```python
from build123d import *

# Parameters (mm, degrees)
SKETCH1_W                    = 50.8
SKETCH1_H                    = 40
BASE_FLANGE1_DEPTH           = 0.635
EDGE_FLANGE1_STRIP_W         = 4.54
EDGE_FLANGE1_STRIP_H         = 0.635
EDGE_FLANGE1_STRIP_CUT_DEPTH = 50.8
EDGE_FLANGE1_DEPTH           = 50.8
SKETCH9_R                    = 8.75
CUT_EXTRUDE1_DEPTH           = 35.48419928
SKETCH10_R                   = 2.65
CUT_EXTRUDE2_DEPTH           = 49.360761212


# Sheet-metal steps are written as plain solids
with BuildPart() as part:
    # Sketch1 → Base-Flange1 (new body)
    with BuildSketch(Plane(origin=(0, 0, 0), x_dir=(0, 0, -1), z_dir=(1, 0, 0))):
        Rectangle(SKETCH1_W, SKETCH1_H)
    extrude(amount=-BASE_FLANGE1_DEPTH)

    # Edge-Flange1 strip (across the edge) → Edge-Flange1 strip cut (cut)
    with BuildSketch(Plane(origin=(-0.635, -20, -25.4), x_dir=(0, 1, 0), z_dir=(0, 0, 1))):
        with Locations((-0.635, -0.3175)):
            Rectangle(EDGE_FLANGE1_STRIP_W, EDGE_FLANGE1_STRIP_H)
    extrude(amount=EDGE_FLANGE1_STRIP_CUT_DEPTH, mode=Mode.SUBTRACT)

    # Edge-Flange1 section (across the edge) → Edge-Flange1 (add)
    with BuildSketch(Plane(origin=(-0.635, -20, -25.4), x_dir=(0, 1, 0), z_dir=(0, 0, 1))):
        with BuildLine():
            Line((0, 1), (0, 11.365))
            Line((0, 11.365), (0.635, 11.365))
            Line((0.635, 11.365), (0.635, 1))
            ThreePointArc((0.635, 1), (0.927893219, 0.292893219), (1.635, 0))
            Line((1.635, 0), (1.635, -0.635))
            ThreePointArc((1.635, -0.635), (0.478880413, -0.156119587), (0, 1))
        make_face()
    extrude(amount=EDGE_FLANGE1_DEPTH)

    # Sketch9 → Cut-Extrude1 (cut, through all)
    with BuildSketch(Plane(origin=(0, 0, 0), x_dir=(0, 0, -1), z_dir=(1, 0, 0))):
        with Locations((0.287892683, 5)):
            Circle(SKETCH9_R)
    extrude(amount=-CUT_EXTRUDE1_DEPTH, mode=Mode.SUBTRACT)

    # Sketch10 → Cut-Extrude2 (cut, through all)
    with BuildSketch(Plane(origin=(0, -19.365, 0), x_dir=(1, 0, 0), z_dir=(0, 1, 0))):
        with Locations(Location((-6.8175, 12, 0), (0, 0, 180))):
            Circle(SKETCH10_R)
        with BuildLine():
            Line((-4.1675, -9.5), (-4.1675, -14.5))
            ThreePointArc((-4.1675, -14.5), (-6.8175, -17.15), (-9.4675, -14.5))
            Line((-9.4675, -14.5), (-9.4675, -9.5))
            ThreePointArc((-9.4675, -9.5), (-6.8175, -6.85), (-4.1675, -9.5))
        make_face()
    extrude(amount=-CUT_EXTRUDE2_DEPTH, mode=Mode.SUBTRACT)


solid = part.part
```
Could you check a few things on this model? Use its own coordinates, in mm. A direction names the side the tool comes from. Give positions to 0.01 mm unless a question says otherwise; leave off trailing zeros. Loops run counter-clockwise (first coordinate to the right, second up) from the corner with the lowest first, then second, coordinate; pieces in that order, holes last. Notation, with made-up numbers: (4, -19) - (14, -19) arc R14 cw to (14, 4) - close; hole circle Ø10 at (13.5, 66.25). An arc over 180 degrees is marked (long way). Answer in a Markdown table with one row per item. Add a question column.
Q1. If we section it at B-B (z = -12): List the corners of the cut face in (x, y) for me (1 decimal), plus the area to 3 significant figures.
Q2. If we section it at D-D (z = -6): List the corners of the cut face in (x, y) for me (3 decimals), plus the area to 3 significant figures.
Q3. We'd pull the mould along Y, two halves only. Please class faces 1 (the face through (-0.31, -0.32, 6.66)), 2 (the face through (-0.47, -19.51, -0.36)), 3 (the face through (-0.635, -3, -5)): +Y half, -Y half, draft (parallel to the pull), parting line (faces both ways), or undercut.
Q4. For pin 1 (5 mm diameter, centred on x = -5, z = -9, fed in from +Y) (3 decimals), with a flat end and sliding along its axis, tell me the tip position at first contact or that it passes through.
Q5. Please list where these lines run through material, in increasing order: L1, parallel to Y at x = -7, z = -18.5 (3 decimals); L2, parallel to X at y = 8.5, z = 10.5 (3 decimals). Write a range as from..to.
Q6. If we section it at C-C (x = -11): List the corners of the cut face in (y, z) for me (3 decimals), plus the area to 3 significant figures.
Q7. If we section it at A-A (y = 5): List the corners of the cut face in (x, z) for me (3 decimals).
Q8. Which directions (+Z, -Z, +X, -X, +Y, -Y) give clear straight access to the entire face, cutting with the end or side of a thin tool? Please do faces 4 (the face through (-6.88, -19.68, 6.85)), 5 (the face through (-7, -19.365, 0)), 6 (the face through (-0.3, 0.1, 25.4)).
The answers:
| question | item | result |
|---|---|---|
| 1 | outline | (-12, -20) - (-9.5, -20) - (-9.5, -19.4) - (-12, -19.4) - close; (-4.2, -20) - (-1.6, -20) arc R1.6 ccw to (0, -18.4) - (0, 20) - (-0.6, 20) - (-0.6, -18.4) arc R1 cw to (-1.6, -19.4) - (-4.2, -19.4) - close |
| 1 | area | 28.9 mm^2 |
| 2 | outline | (-12, -20) - (-1.635, -20) arc R1.635 ccw to (0, -18.365) - (0, -1.628) - (-0.635, -1.628) - (-0.635, -18.365) arc R1 cw to (-1.635, -19.365) - (-12, -19.365) - close; (-0.635, 11.628) - (0, 11.628) - (0, 20) - (-0.635, 20) - close |
| 2 | area | 23.8 mm^2 |
| 3 | face 1 | undercut |
| 3 | face 2 | -Y half |
| 3 | face 3 | draft |
| 4 | pin 1 | stops at y = -19.365 |
| 5 | L1 | y = -20..-19.365 |
| 5 | L2 | x = -0.635..0 |
| 6 | outline | (-20, -25.4) - (-19.365, -25.4) - (-19.365, 25.4) - (-20, 25.4) - close |
| 6 | area | 32.3 mm^2 |
| 7 | outline | (-0.635, -25.4) - (0, -25.4) - (0, -9.038) - (-0.635, -9.038) - close; (-0.635, 8.462) - (0, 8.462) - (0, 25.4) - (-0.635, 25.4) - close |
| 8 | face 4 | +Y, -Y |
| 8 | face 5 | +Z, -Z, -X, +Y |
| 8 | face 6 | +Z, +X, -X, +Y, -Y |
